Input: part model. Units: mm. Frame: model coordinates. Face numbers are marked on the shaded views. Coordinates: 2 decimals unless noted, no trailing zeros. Order: outer loops, then holes, each group sorted by start corner. A loop starts at its lowest first (then second) coordinate and runs counter-clockwise, first axis right, second up.
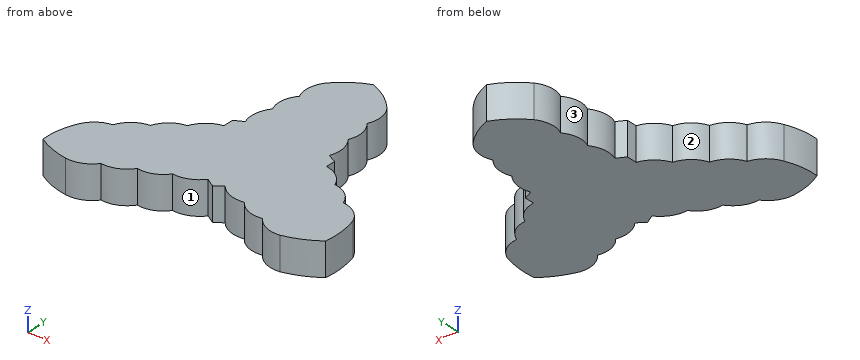
from build123d import *

# Parameters (mm, degrees)
F1_DEPTH = 7.9375


# Not quite as in the source:
# - a length typed as a fraction of an inch, garbled in the dataset ("3 / 203.2 mm" for 3/8 in), is restored


with BuildPart() as f1:
    # F0 (on Top) → F1 (new body)
    with BuildSketch(Plane.XY):
        with BuildLine():
            ThreePointArc((-0.0986067535, 34.0497419238), (-4.0682176485, 31.9659465467), (-7.4162920937, 28.9842672646))
            ThreePointArc((-7.4162920937, 28.9842672646), (-8.8119305122, 25.5953281623), (-8.2258973271, 21.977417171))
            ThreePointArc((-8.2258973271, 21.977417171), (-9.7181261566, 18.698842434), (-9.2097157612, 15.1327075437))
            ThreePointArc((-9.2097157612, 15.1327075437), (-10.6205392688, 11.8246856933), (-10.2093555033, 8.2519613206))
            Line((-10.2093555033, 8.2519613206), (-12.369341217, 7.1464567445))
            Line((-12.369341217, 7.1464567445), (-12.369341217, 4.6386048198))
            Line((-12.369341217, 4.6386048198), (-12.369341217, 4.5682978211))
            ThreePointArc((-12.369341217, 4.5682978211), (-15.5930977879, 3.1185654947), (-17.7027139134, 0.2823972963))
            ThreePointArc((-17.7027139134, 0.2823972963), (-21.0452825194, -1.0603738309), (-23.1384971151, -3.9919692741))
            ThreePointArc((-23.1384971151, -3.9919692741), (-26.5647165348, -5.2934051439), (-28.80180468, -8.19653302))
            ThreePointArc((-28.80180468, -8.19653302), (-32.1117440701, -9.5846599904), (-34.254974256, -12.4637500588))
            ThreePointArc((-34.254974256, -12.4637500588), (-35.4454588739, -16.4293701566), (-35.6585793197, -20.564340055))
            ThreePointArc((-35.6585793197, -20.564340055), (-31.9389059128, -22.4150036937), (-27.9142765499, -23.4461606411))
            ThreePointArc((-27.9142765499, -23.4461606411), (-24.3492963179, -23.0296138883), (-21.4921734029, -20.8571857766))
            ThreePointArc((-21.4921734029, -20.8571857766), (-17.8594468391, -20.3713745504), (-15.0192606046, -18.054899429))
            ThreePointArc((-15.0192606046, -18.054899429), (-11.4338171794, -17.7079201351), (-8.5996589687, -15.484556372))
            ThreePointArc((-8.5996589687, -15.484556372), (-5.0294162563, -15.0523544446), (-2.1409380715, -12.9098966718))
            Line((-2.1409380715, -12.9098966718), (0, -14.2561570176))
            Line((0, -14.2561570176), (1.9696742658, -12.9098966718))
            ThreePointArc((1.9696742658, -12.9098966718), (4.9392756736, -15.0084468105), (8.560301624, -15.3410370587))
            ThreePointArc((8.560301624, -15.3410370587), (11.3944598347, -17.5644008218), (14.9799032599, -17.9113801157))
            ThreePointArc((14.9799032599, -17.9113801157), (17.8200894944, -20.2278552371), (21.4528160582, -20.7136664634))
            ThreePointArc((21.4528160582, -20.7136664634), (25.6558468929, -19.2922500665), (29.4813849032, -17.0447733253))
            ThreePointArc((29.4813849032, -17.0447733253), (29.5836204245, -12.511977875), (28.7624473353, -8.0530137067))
            ThreePointArc((28.7624473353, -8.0530137067), (26.5253591901, -5.1498858306), (23.0991397704, -3.8484499608))
            ThreePointArc((23.0991397704, -3.8484499608), (21.0059251747, -0.9168545176), (17.6633565687, 0.4259166096))
            ThreePointArc((17.6633565687, 0.4259166096), (15.4847616458, 3.3168082822), (12.1560195839, 4.739132713))
            Line((12.1560195839, 4.739132713), (12.1560195839, 7.1464567445))
            Line((12.1560195839, 7.1464567445), (9.9960338703, 8.2519613206))
            ThreePointArc((9.9960338703, 8.2519613206), (10.4072176357, 11.8246856933), (8.9963941282, 15.1327075437))
            ThreePointArc((8.9963941282, 15.1327075437), (9.5048045235, 18.698842434), (8.012575694, 21.977417171))
            ThreePointArc((8.012575694, 21.977417171), (8.5986088792, 25.5953281623), (7.2029704606, 28.9842672646))
            ThreePointArc((7.2029704606, 28.9842672646), (3.8655773676, 31.9687453881), (-0.0986067535, 34.0497419238))
        make_face()
    extrude(amount=F1_DEPTH)


solid = f1.part
Item 1: Pin query (flat end, axial travel): pin 1 Ø6 at (x, y) = (-16.5, 12) entering from +Z; pin 2 Ø1 at (y, z) = (-14, 5.5) entering from -X; pin 3 Ø1.3 at (y, z) = (6.5, 2) entering from -X; pin 4 Ø2 at (y, z) = (1.5, 6) entering from +X. Return the tip coordinate at first contact, or that it passes through.
Response values:
pin 1: passes through
pin 2: stops at x = -35
pin 3: stops at x = -12.37
pin 4: stops at x = 17.63
Item 2: Cut plane B-B on x = -5.5. Return loops of the section in (y, z), then the cut area to 3 significant figures.
Response values:
outline: (-15.22, 0) - (30.87, 0) - (30.87, 7.94) - (-15.22, 7.94) - close
area: 366 mm2
Item 3: Cut plane C-C on y = 19. Return loops of the section in (x, z).
Response values:
outline: (-9.67, 0) - (9.45, 0) - (9.45, 7.94) - (-9.67, 7.94) - close
Item 4: Ray query, probe 1 along X at (y, z) = (7, 7); probe 2 along Y at (x, z) = (-14, 2.25); probe 3 along X at (y, z) = (-8, 5.25). Return the intervals inside material, ascending.
Response values:
probe 1: x = -12.37 to 12.16
probe 2: y = -18.17 to 4.08
probe 3: x = -28.72 to 28.74
Item 5: Draft query along Y for the marked faces 1, 2 and 3. Return one class per face: pulls with the +Y half, pulls with the -Y half, needs draft (parallel to the pull), parting line crosses it, or undercut.
Response values:
face 1: pulls with the -Y half
face 2: pulls with the +Y half
face 3: undercut
